Input: part model. Units: mm. Frame: model coordinates. Face numbers are marked on the shaded views. Coordinates: 2 decimals unless noted, no trailing zeros. Write each loop counter-clockwise with the first axis right and the second up, starting at its lowest first coordinate (ties: lowest second). Pieces come first, ordered by that corner, then holes. Notation, with made-up numbers: (34.5, 48.25) -> (60.5, 48.25) arc R25 ccw to (60.5, 70.25) -> close; hole circle Ø10 at (41.5, -39). An arc over 180 degrees is marked (long way). Use one line per item in the form item = value. Start each with the question number.
(1) Pull-direction query (Z, two-part tool) for the marked faces 1, 2 and 3; classes: released by +Z, released by -Z, zero draft, split by the parting line, or undercut.
(2) Cut plane B-B on z = -51.5. Return the cut outline in (x, y), plus the area to 3 significant figures.
(3) Ray query, line 1 along Z through (x, y) = (0, 24.5); line 2 along X through (y, z) = (24, -55); line 3 along Y through (x, z) = (-6, -82.5). Return the intervals inside material, ascending.
(4) Cut plane C-C on y = 24. Return the cut outline in (x, z), plus the area to 3 significant figures.
(5) Cut plane A-A on x = 0. Return the cut outline in (y, z), plus the area to 3 significant figures.
(6) First-contact query: pin 1 (2 mm diameter, centred on x = 12.5, z = -26, fed in from +Y). Flat tip, straight axial feed; report the tip coordinate or a pass-through.
(7) Cut plane D-D on x = -14. Return the cut outline in (y, z).
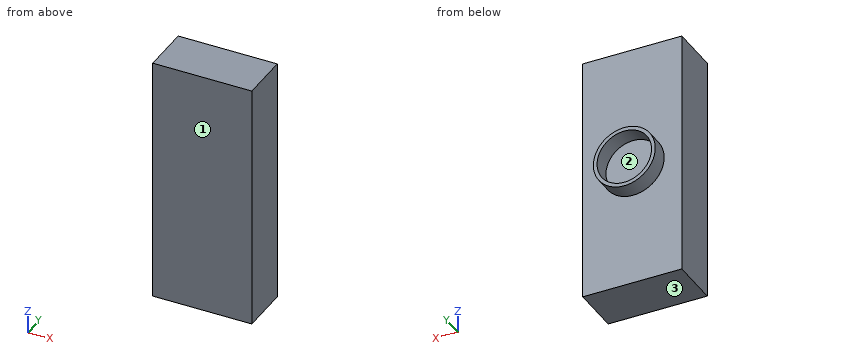
Autodesk Inventor part; units mm, degrees
ref_plane "YZ Plane" through (0, 0, 0) normal (1, 0, 0) x (0, 1, 0)
ref_plane "XZ Plane" through (0, 0, 0) normal (0, 1, 0) x (-1, 0, 0)
ref_plane "XY Plane" through (0, 0, 0) normal (0, 0, 1) x (1, 0, 0)
sketch "Esboço1" plane through (0, 0, 0) normal (0, 1, 0) x (-1, 0, 0)
  line L0 (19.6154, -5.2564) -> (-20.3846, -5.2564)
  line L1 (-20.3846, -5.2564) -> (-20.3846, -105.2564)
  line L2 (-20.3846, -105.2564) -> (19.6154, -105.2564)
  line L3 (19.6154, -105.2564) -> (19.6154, -5.2564)
  point P0 (0, 0)
  dimension "d0" = 40
  dimension "d4" = 100
extrude "Extrusão1" add sketch "Esboço1" along normal blind 20
sketch "Esboço2" plane through (0, 20, 0) normal (0, 1, 0) x (1, 0, 0)
  circle A0 centre (0, 55.2564) radius 12.5
  circle A1 centre (0, 55.2564) radius 11
  line L0 (20.3846, 105.2564) -> (-19.6154, 105.2564)
  point P0 (0, 0)
  dimension "d11" = 22
  dimension "d12" = 25
  dimension "d13" = 50
extrude "Extrusão2" add sketch "Esboço2" along normal blind 7
sketch "Esboço3" plane through (0, 0, 0) normal (0, -1, 0) x (1, 0, 0)
  circle A0 centre (0.3846, -25.2576) radius 2.5
  circle A1 centre (0, -85.2564) radius 2.5
  line L0 (20.3846, -105.2564) -> (-19.6154, -105.2564)
  line L1 (20.3846, -5.2564) -> (20.3846, -105.2564)
  point P0 (0, 0)
  dimension "d16" = 5
  dimension "d17" = 5
  dimension "d18" = 60
  dimension "d19" = 20
  dimension "d20" = 20
properties part number "Suporte para estrutura" material "ABS plástico"
Values:
q1.face_1 = zero draft
q1.face_2 = undercut
q1.face_3 = released by -Z
q2.outline = (-19.62, 0) -> (20.38, 0) -> (20.38, 20) -> (11.92, 20) -> (11.92, 27) -> (10.34, 27) -> (10.34, 20) -> (-10.34, 20) -> (-10.34, 27) -> (-11.92, 27) -> (-11.92, 20) -> (-19.62, 20) -> close
q2.area = 822 mm2
q3.line_1 = -67.76 to -66.26, -44.26 to -42.76
q3.line_2 = -12.5 to -11, 11 to 12.5
q3.line_3 = 0 to 20
q4.outline = circle Ø25 at (0, -55.26); hole circle Ø22 at (0, -55.26)
q4.area = 111 mm2
q5.outline = (0, -105.26) -> (20, -105.26) -> (20, -67.76) -> (27, -67.76) -> (27, -66.26) -> (20, -66.26) -> (20, -44.26) -> (27, -44.26) -> (27, -42.76) -> (20, -42.76) -> (20, -5.26) -> (0, -5.26) -> close
q5.area = 2,020 mm2
q6.pin_1 = 20
q7.outline = (0, -105.26) -> (20, -105.26) -> (20, -5.26) -> (0, -5.26) -> close
